```python
from build123d import *

# Parameters (mm, degrees)
F1_DEPTH  = 32
F3_DEPTH  = 19
F5_DEPTH  = 19
F7_DEPTH  = 25
F8_R      = 5.506936
F9_DEPTH  = 13.001
F10_R     = 6.5
F11_DEPTH = 88.001


with BuildPart() as f1:
    # F0 (on Front) → F1 (new body)
    with BuildSketch(Plane.XZ):
        Polygon((-25, 13), (-25, 0), (14, 0), (14, 17), (49, 17), (49, 0), (88, 0), (88, 13), (63, 13), (63, 64), (44, 64), (44, 30), (19, 30), (19, 64), (0, 64), (0, 13), align=None)
    extrude(amount=F1_DEPTH)

    # F2 (on face) → F3 (join)
    with BuildSketch(Plane.YZ.offset(63)):
        with BuildLine():
            Line((-32, 64), (0, 64))
            ThreePointArc((0, 64), (-16, 67.871235), (-32, 64))
        make_face()
    extrude(amount=-F3_DEPTH)

    # F4 (on face) → F5 (join)
    with BuildSketch(Plane(origin=(0, 0, 0), x_dir=(0, -1, 0), z_dir=(-1, 0, 0))):
        with BuildLine():
            Line((0, 64), (32, 64))
            ThreePointArc((32, 64), (16, 67.871235), (0, 64))
        make_face()
    extrude(amount=-F5_DEPTH)

    # F6 (on face) → F7 (cut)
    with BuildSketch(Plane.XY.offset(13)):
        Polygon((-25, -10), (-15, 0), (-25, 0), align=None)
        Polygon((-25, -22), (-25, -32), (-15, -32), align=None)
    extrude(amount=-F7_DEPTH, mode=Mode.SUBTRACT)

    # F8 (on face) → F9 (cut, through all)
    with BuildSketch(Plane.XY.offset(13)):
        with Locations((75, -16)):
            Circle(F8_R)
        Polygon((88, 0), (78, 0), (88, -10), align=None)
        Polygon((88, -32), (88, -22), (78, -32), align=None)
        with Locations((-12, -16)):
            Circle(F8_R)
    extrude(amount=-F9_DEPTH, mode=Mode.SUBTRACT)

    # F10 (on face) → F11 (cut, through all)
    with BuildSketch(Plane.YZ.offset(63)):
        with Locations((-16, 49.871235)):
            Circle(F10_R)
    extrude(amount=-F11_DEPTH, mode=Mode.SUBTRACT)


solid = f1.part
```
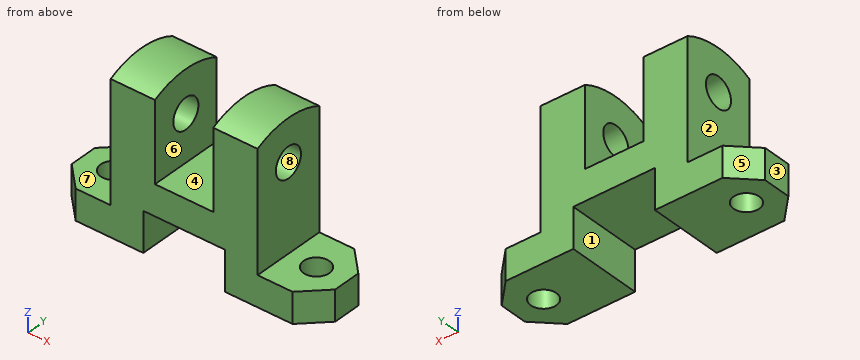
Geometry: final body of the model. Coordinates: model frame, mm. Face numbers are marked on the shaded views. A direction names the side the tool comes from. Give positions to 0.01 mm unless a question says otherwise; leave off trailing zeros. Write each loop counter-clockwise with the first axis right and the second up, starting at its lowest first coordinate (ties: lowest second). Pieces come first, ordered by that corner, then holes.
1. Line query: probe 1 along X at (y, z) = (-19, 36.5); probe 2 along Y at (x, z) = (-12, 4); probe 3 along Z at (x, y) = (51.75, -16). Output: solid intervals per line, ascending.
2. Draft query along Z for the marked faces 6, 7 and 8. Return one class per face: released by +Z, released by -Z, zero draft, split by the parting line, or undercut.
3. Section query A-A, the plane x = -12. Return loops of the section in (y, z).
4. Reachability of the marked faces 1, 2, 3, 4 and 5 from +Z, -Z, +X, -X, +Y, -Y: full face, straight path, thin tool, end or side. Return the list, or none.
5. Section query D-D, the plane z = 48. Return loops of the section in (x, y).
6. Section query C-C, the plane y = -16. Count the separate pieces of the cut face and the enclosed holes in it, then the cut area to 3 significant figures.
7. Section query B-B, the plane z = 39. Return loops of the section in (x, y).
8. Pin query (flat end, axial travel): P1, Ø1.5, axis at y = -28.5, z = 9.5, coming from the -X side; P2, Ø5, axis at x = 40.5, y = -5, coming from the +Z side; P3, Ø3, axis at y = -26, z = 53, coming from the -X side. Return the tip coordinate at first contact, or that it passes through.
Computed:
1. probe 1: x = 0 to 19, 44 to 63
1. probe 2: y = -32 to -21.51, -10.49 to 0
1. probe 3: z = 0 to 43.37, 56.37 to 67.87
2. face 6: zero draft
2. face 7: released by +Z
2. face 8: undercut
3. outline: (-32, 0) - (-21.51, 0) - (-21.51, 13) - (-32, 13) - close; (-10.49, 0) - (0, 0) - (0, 13) - (-10.49, 13) - close
4. face 1: -Z, +Y, -Y
4. face 2: +Z, -X, +Y, -Y
4. face 3: +Z, -Z, -X, +Y, -Y
4. face 4: +Z, +Y, -Y
4. face 5: +Z, -Z, -X, +Y
5. outline: (0, -32) - (19, -32) - (19, -22.22) - (0, -22.22) - close; (0, -9.78) - (19, -9.78) - (19, 0) - (0, 0) - close; (44, -32) - (63, -32) - (63, -22.22) - (44, -22.22) - close; (44, -9.78) - (63, -9.78) - (63, 0) - (44, 0) - close
6. separate pieces: 5
6. enclosed holes: 0
6. area: 2,600 mm2
7. outline: (0, -32) - (19, -32) - (19, 0) - (0, 0) - close; (44, -32) - (63, -32) - (63, 0) - (44, 0) - close
8. P1: stops at x = -19.25
8. P2: stops at z = 30
8. P3: stops at x = 0
